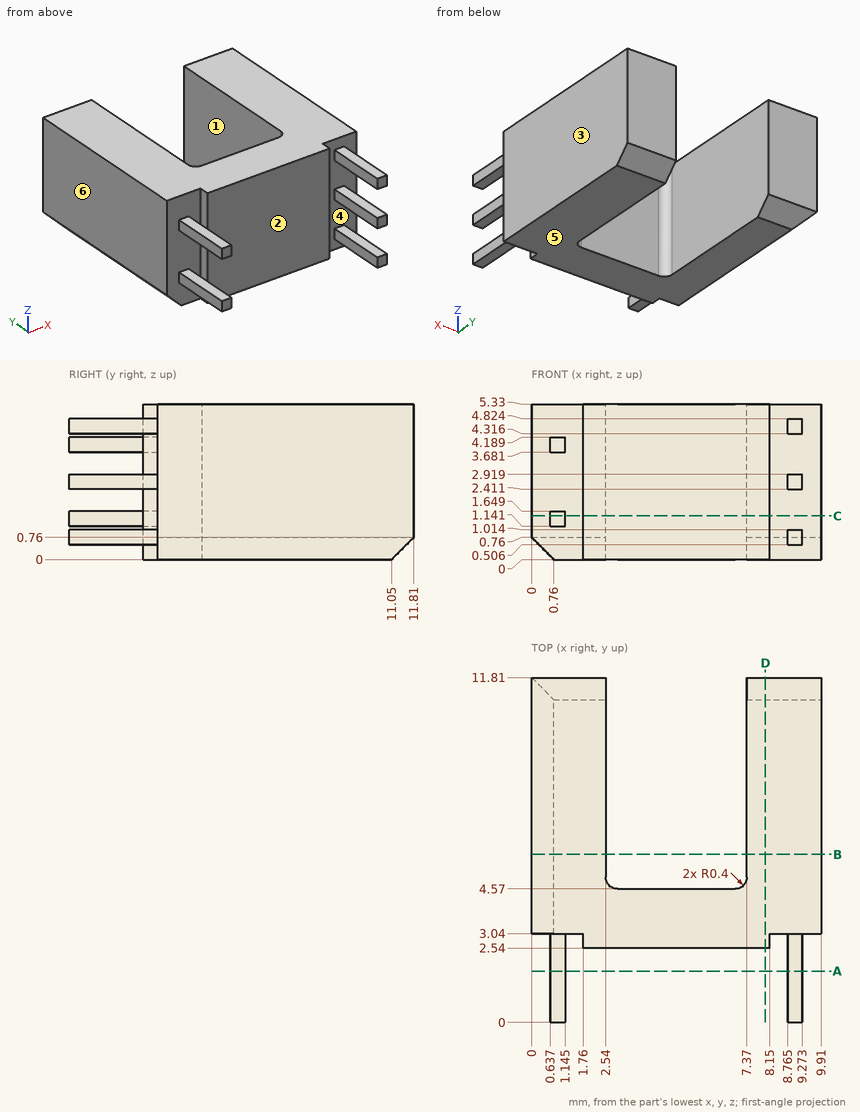
For this review, use the dimensioned drawing (mm, ordinates from the lowest corner) and the shaded views. A direction names the side the tool comes from. Round coordinates to 2 decimals unless told otherwise and drop trailing zeros. Loops run counter-clockwise (first coordinate to the right, second up) from the corner with the lowest first, then second, coordinate; pieces in that order, holes last. Notation, with made-up numbers: (-9.75, 43.5) -> (37.25, 43.5) arc R27 ccw to (37.25, 71.5) -> close; hole circle Ø7 at (29.5, -29.5). An arc over 180 degrees is marked (long way). Write item = value, one per line. Start each with the question number.
Item 1: Take a section at C-C on z = 1.5. Give the boundary of the cut face in (x, y) (3 decimals).
Item 2: Take a section at B-B on y = 5.75. Give the boundary of the cut face in (x, z), plus the area to 3 significant figures.
Item 3: Mouldability with a two-part tool opening along Z and no side actions: class the marked faces 4, 5 and 6 as released by +Z, released by -Z, zero draft, split by the parting line, or undercut.
Item 4: To check wall thickness, follow L1, parallel to X at y = 8, z = 5.1; L2, parallel to Y at x = 2, z = 2.3; L3, parallel to Y at x = 5.75, z = 2.7. State the ranges of each line that lie inside material, in increasing order.
Item 5: Take a section at D-D on x = 8. Give the boundary of the cut face in (y, z).
Item 6: Take a section at A-A on y = 1.75. Give the boundary of the cut face in (x, z) (3 decimals).
Item 7: Insertion check: pin 1 (1.4 mm diameter, centred on x = 0.5, z = 2, fed in from -Y). The pin has a flat end and moves straight along its axis. Give the tip position at first contact, or say it passes through.
Item 8: For the marked faces 1, 2 and 3, list the 3-axis set-ups (+Z, -Z, +X, -X, +Y, -Y) from which the entire face can be reached by the end or side of a thin tool; tool diameter is ignored.
Result:
q1.outline = (0, 3.04) -> (0.637, 3.04) -> (0.637, 0) -> (1.145, 0) -> (1.145, 3.04) -> (1.76, 3.04) -> (1.76, 2.54) -> (8.15, 2.54) -> (8.15, 3.04) -> (9.91, 3.04) -> (9.91, 11.81) -> (7.37, 11.81) -> (7.37, 4.97) arc R0.4 cw to (6.97, 4.57) -> (2.94, 4.57) arc R0.4 cw to (2.54, 4.97) -> (2.54, 11.81) -> (0, 11.81) -> close
q2.outline = (0, 0.76) -> (0.76, 0) -> (2.54, 0) -> (2.54, 5.33) -> (0, 5.33) -> close; (7.37, 0) -> (9.91, 0) -> (9.91, 5.33) -> (7.37, 5.33) -> close
q2.area = 26.8 mm²
q3.face_4 = undercut
q3.face_5 = released by -Z
q3.face_6 = zero draft
q4.L1 = 0 to 2.54, 7.37 to 9.91
q4.L2 = 2.54 to 11.81
q4.L3 = 2.54 to 4.57
q5.outline = (2.54, 0) -> (11.05, 0) -> (11.81, 0.76) -> (11.81, 5.33) -> (2.54, 5.33) -> close
q6.outline = (0.637, 1.141) -> (1.145, 1.141) -> (1.145, 1.649) -> (0.637, 1.649) -> close; (0.637, 3.681) -> (1.145, 3.681) -> (1.145, 4.189) -> (0.637, 4.189) -> close; (8.765, 0.506) -> (9.273, 0.506) -> (9.273, 1.014) -> (8.765, 1.014) -> close; (8.765, 2.411) -> (9.273, 2.411) -> (9.273, 2.919) -> (8.765, 2.919) -> close; (8.765, 4.316) -> (9.273, 4.316) -> (9.273, 4.824) -> (8.765, 4.824) -> close
q7.pin_1 = 0
q8.face_1 = +Z, -Z, +Y
q8.face_2 = +Z, -Z, -Y
q8.face_3 = +Z, -Z, +X, +Y, -Y
